Geometry check sheet. Reference: the model listing, model coordinates, mm. A direction names the side the tool comes from. Coordinates: 2 decimals unless noted, no trailing zeros. Write each loop counter-clockwise with the first axis right and the second up, starting at its lowest first coordinate (ties: lowest second). Pieces come first, ordered by that corner, then holes. Notation, with made-up numbers: (62.25, -22) -> (92.25, -22) arc R33 ccw to (92.25, 9) -> close; hole circle Ø11 at (51.25, -8.75). An arc over 180 degrees is marked (long way). Answer as CSV lines item,"result".
```python
from build123d import *

# Parameters (mm, degrees)
F1_R     = 7.9375
F2_DEPTH = 107.95
F0_R     = 12.7
F3_DEPTH = 57.15
F5_DEPTH = 1.5875


with BuildPart() as f2:
    # F1 (on Right) → F2 (new body)
    with BuildSketch(Plane.YZ):
        Circle(F1_R)
    extrude(amount=F2_DEPTH)

    # F0 (on Front) → F3 (join, symmetric)
    with BuildSketch(Plane.XZ):
        Circle(F0_R)
    extrude(amount=F3_DEPTH, both=True)

    # F4 (on Front) → F5 (join, symmetric)
    with BuildSketch(Plane.XZ):
        Polygon((-6.35, 6.35), (0, 6.35), (6.35, 6.35), (6.35, 44.45), (-6.35, 44.45), align=None)
    extrude(amount=F5_DEPTH, both=True)


solid = f2.part
```
Item 1: Cross-section at B-B, the plane y = 0. Record the cut outline in (x, z).
Responses:
outline,"(-6.35, 11) arc R12.7 ccw (long way) to (9.91, -7.94) -> (107.95, -7.94) -> (107.95, 7.94) -> (9.91, 7.94) arc R12.7 ccw to (6.35, 11) -> (6.35, 44.45) -> (-6.35, 44.45) -> close"
Item 2: Cross-section at A-A, the plane z = 0. Record the cut outline in (x, y), plus the area to 3 significant figures.
Responses:
outline,"(-12.7, -57.15) -> (12.7, -57.15) -> (12.7, -7.94) -> (107.95, -7.94) -> (107.95, 7.94) -> (12.7, 7.94) -> (12.7, 57.15) -> (-12.7, 57.15) -> close"
area,"4,420 mm2"
Item 3: Cross-section at C-C, the plane x = 25.5. Record the cut outline in (y, z) (1 decimal), plus the area to 3 significant figures.
Responses:
outline,"circle Ø15.9 at (0, 0)"
area,"198 mm2"
Item 4: Cross-section at D-D, the plane z = 32. Record the cut outline in (x, y).
Responses:
outline,"(-6.35, -1.59) -> (6.35, -1.59) -> (6.35, 1.59) -> (-6.35, 1.59) -> close"
Item 5: Set-up check for faces 1 (the flat face through (6.35, 0, 27)), 2 (the cylindrical face through (-10.1, -0.8, -7.7)), 3 (the flat face through (-6.35, 0, 28)), 4 (the cylindrical face through (58.25, -1.72, -7.75)): record each of +Z, -Z, +X, -X, +Y, -Y from which the full face is reachable in a straight line by a thin tool's end or side.
Responses:
face 1,"+Z, +X, +Y, -Y"
face 2,"none"
face 3,"+Z, -X, +Y, -Y"
face 4,"+X"
Item 6: Thickness scan on probe 1 along Y at (x, z) = (4.5, 34); probe 2 along X at (y, z) = (0.5, 13); probe 3 along Z at (x, y) = (47.5, -3.5). Record the ranges inside material, lowest first.
Responses:
probe 1,"y = -1.59 to 1.59"
probe 2,"x = -6.35 to 6.35"
probe 3,"z = -7.12 to 7.12"
Item 7: Depth check by flat-ended pin: pin 1 Ø4 at (x, z) = (-3, 20.5) entering from +Y; pin 2 Ø10 at (y, z) = (24, 12) entering from +X; pin 3 Ø2 at (y, z) = (3, 1.5) entering from -X. Enter the tip coordinate at first touch or a pass-through.
Responses:
pin 1,"stops at y = 1.59"
pin 2,"stops at x = 10.6"
pin 3,"stops at x = -12.69"
